```python
from build123d import *

# Parameters (mm, degrees)
F0_R     = 7.493
F1_DEPTH = 2
F2_R     = 1.1049
F3_DEPTH = 25.4
F4_R     = 0.254


with BuildPart() as f1:
    # F0 (on Top) → F1 (new body)
    with BuildSketch(Plane.XY):
        Circle(F0_R)
    extrude(amount=F1_DEPTH)

    # F2 (on face) → F3 (cut)
    with BuildSketch(Plane.XY.offset(2)):
        with Locations((-4.407408, 0)):
            Circle(F2_R)
        Circle(F2_R)
        with Locations((0, 4.407408)):
            Circle(F2_R)
        with Locations((4.407408, 0)):
            Circle(F2_R)
        with Locations((0, -4.407408)):
            Circle(F2_R)
    extrude(amount=-F3_DEPTH, mode=Mode.SUBTRACT)

    # F4
    f4_edges = [f1.edges().sort_by_distance(p)[0] for p in [
        (-7.493, 0, 2),
        (-7.493, 0, 0),
    ]]
    fillet(f4_edges, radius=F4_R)


solid = f1.part
```
Source: CAD feature listing. Evaluate the final solid. Frame: model axes, mm. Round coordinates to 2 decimals unless told otherwise and drop trailing zeros. Write each loop counter-clockwise with the first axis right and the second up, starting at its lowest first coordinate (ties: lowest second). Pieces come first, ordered by that corner, then holes. Notation, with made-up numbers: M 47.25,-34 L 81.25,-34 A31 cw 81.25,-1 Z; hole C 53,59.5 d5. An arc over 180 degrees is marked long. Answer as a JSON object with one key per item and string values. Group by question number.
(1) First-contact query: pin 1 (1 mm diameter, centred on x = 3, z = 0.5, fed in from -Y). Flat tip, straight axial feed; report the tip coordinate or a pass-through.
(2) Ray query, line 1 (Y direction, x = 0, z = 0.45); line 2 (Y direction, x = -1, z = 0.6); line 3 (Y direction, x = 5, z = 1.05). Return the intervals inside material, ascending. Write a range as [from, to].
(3) Section query A-A on y = 0. Output: boundary loops of the cut face in (x, z), then the cut area to 3 significant figures.
(4) Mould query, pull axis Y, two halves, no side actions, for faces 1 (the cylindrical face through (-0.98, 7.43, 0.99)), 2 (the flat face through (2, 0, 2)), 3 (the cylindrical face through (-0.14, -3.31, 1.01)). Classes: +Y half, -Y half, draft (parallel to the pull), parting line (faces both ways), or undercut.
(5) Section query C-C on z = 1.3. Output: boundary loops of the cut face in (x, y).
Computed values:
{
 "1": {"pin 1": "y = -7.06"},
 "2": {"line 1": "[-7.49, -5.51], [-3.3, -1.1], [1.1, 3.3], [5.51, 7.49]", "line 2": "[-7.43, -4.88], [-3.94, -0.47], [0.47, 3.94], [4.88, 7.43]", "line 3": "[-5.58, -0.93], [0.93, 5.58]"},
 "3": {"outline": "M -7.49,0.25 A0.25 ccw -7.24,0 L -5.51,0 L -5.51,2 L -7.24,2 A0.25 ccw -7.49,1.75 Z; M -3.3,0 L -1.1,0 L -1.1,2 L -3.3,2 Z; M 1.1,0 L 3.3,0 L 3.3,2 L 1.1,2 Z; M 5.51,0 L 7.24,0 A0.25 ccw 7.49,0.25 L 7.49,1.75 A0.25 ccw 7.24,2 L 5.51,2 Z", "area": "16.7 mm^2"},
 "4": {"face 1": "parting line", "face 2": "draft", "face 3": "undercut"},
 "5": {"outline": "C 0,0 d14.99; hole C -4.41,0 d2.21; hole C 0,-4.41 d2.21; hole C 0,0 d2.21; hole C 0,4.41 d2.21; hole C 4.41,0 d2.21"}
}
